Source: three-view drawing plus pictorial views. Frame: mm from the lowest corner of the part. Give positions to 0.01 mm unless a question says otherwise; leave off trailing zeros. Loops run counter-clockwise (first coordinate to the right, second up) from the corner with the lowest first, then second, coordinate; pieces in that order, holes last. Notation, with made-up numbers: (54.5, -9.75) - (100.5, -9.75) arc R17 ccw to (100.5, 16.25) - close; hole circle Ø4 at (77.5, 14). An arc over 180 degrees is marked (long way). Answer as a JSON object with one key per item and string values.
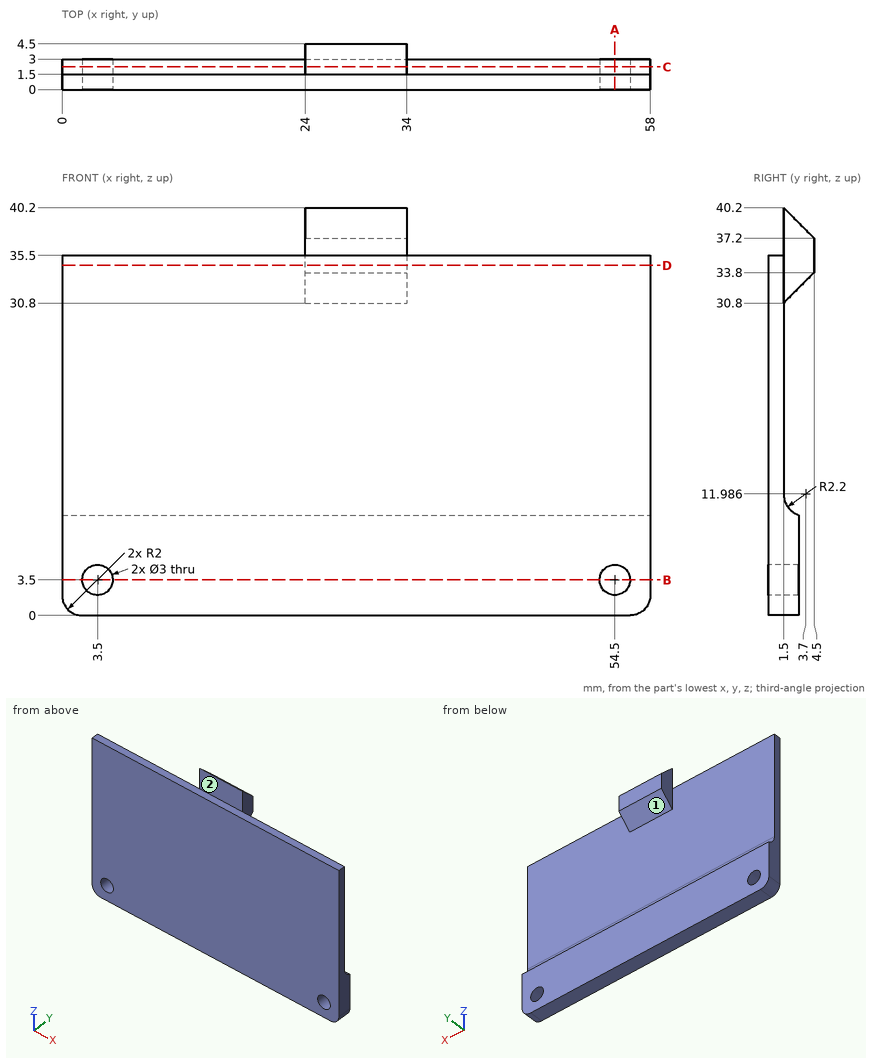
Item 1: Material intervals for line 1 (X direction, y = 1.1, z = 3.5); line 2 (Y direction, x = 21.5, z = 9); line 3 (Y direction, x = 45, z = 19), sorted ascending. Write a range as [from, to].
Geometry check:
{"line 1": "x = [0, 2], [5, 53], [56, 58]", "line 2": "y = [0, 3]", "line 3": "y = [0, 1.5]"}
Item 2: Cut plane C-C (y = 2.25). Return loops of the section in (x, z), then the cut area to 3 significant figures.
Geometry check:
{"outline": "(0, 2) arc R2 ccw to (2, 0) - (56, 0) arc R2 ccw to (58, 2) - (58, 10.33) - (0, 10.33) - close; (24, 31.55) - (34, 31.55) - (34, 39.45) - (24, 39.45) - close; hole circle Ø3 at (3.5, 3.5); hole circle Ø3 at (54.5, 3.5)", "area": "662 mm2"}
Item 3: Mould query, pull axis Z, two halves, no side actions, for the marked faces 1 and 2. Classes: released by +Z, released by -Z, zero draft, split by the parting line, or undercut.
Geometry check:
{"face 1": "undercut", "face 2": "zero draft"}
Item 4: Cut plane D-D (z = 34.5). Return loops of the section in (x, y), then the cut area to 3 significant figures.
Geometry check:
{"outline": "(0, 0) - (58, 0) - (58, 1.5) - (34, 1.5) - (34, 4.5) - (24, 4.5) - (24, 1.5) - (0, 1.5) - close", "area": "117 mm2"}
Item 5: Cut plane B-B (z = 3.5). Return loops of the section in (x, y), then the cut area to 3 significant figures.
Geometry check:
{"outline": "(0, 0) - (2, 0) - (2, 3) - (0, 3) - close; (5, 0) - (53, 0) - (53, 3) - (5, 3) - close; (56, 0) - (58, 0) - (58, 3) - (56, 3) - close", "area": "156 mm2"}
Item 6: Cut plane A-A (x = 54.5). Return loops of the section in (y, z) (1 decimal).
Geometry check:
{"outline": "(0, 0) - (3, 0) - (3, 2) - (0, 2) - close; (0, 5) - (3, 5) - (3, 9.9) arc R2.2 cw to (1.5, 12) - (1.5, 35.5) - (0, 35.5) - close"}
Item 7: Contact query for flat-ended pins moving along their axis: P1, Ø1, axis at y = 2, z = 36, coming from the -X side; P2, Ø3.5, axis at x = 54.5, z = 3.5, coming from the +Y side; P3, Ø7, axis at x = 20, z = 26.5, coming from the +Y side. Output: stop coordinate, or through.
Geometry check:
{"P1": "stops at x = 24", "P2": "stops at y = 3", "P3": "stops at y = 1.5"}
